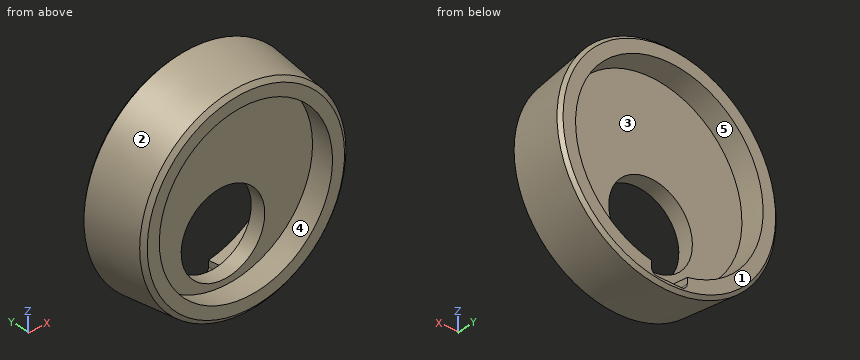
from build123d import *
from OCP.BRepFilletAPI import BRepFilletAPI_MakeChamfer

# Parameters (mm, degrees)
CUT_EXTRUDE1_DEPTH = 28.123421613
SKETCH3_R          = 2
CUT_EXTRUDE2_DEPTH = 2
SKETCH8_R          = 25.2248299
CUT_EXTRUDE4_DEPTH = 12
SKETCH11_R         = 7
CUT_EXTRUDE6_DEPTH = 27.946613887
CUT_EXTRUDE7_DEPTH = 3.6
CHAMFER1_SIZE      = 0.6
CHAMFER1_SIZE2     = 0.68091755
CHAMFER1_SIZE2_2   = 0.542425845


with BuildPart() as part:
    # Sketch1 → Revolve1 (revolve)
    with BuildSketch(Plane.XY, mode=Mode.PRIVATE) as revolve1_sk:
        Polygon((0, 0), (-17.2, 0), (-15.1, -12), (0, -12), align=None)
    revolve(revolve1_sk.sketch.rotate(Axis((0, 0, 0), (0, -1, 0)), 270), axis=Axis((0, 0, 0), (0, -1, 0)))

    # Sketch2 → Cut-Extrude1 (cut, through all)
    with BuildSketch(Plane(origin=(0, 0, 0), x_dir=(1, 0, 0), z_dir=(0, 1, 0))):
        with BuildLine():
            Line((-9.1, -5.8), (-7.3, -5.8))
            Line((-7.3, -5.8), (-7.3, -10.756858277))
            ThreePointArc((-7.3, -10.756858277), (0, -13), (7.3, -10.756858277))
            Line((7.3, -10.756858277), (7.3, -5.8))
            Line((7.3, -5.8), (9.1, -5.8))
            Line((9.1, -5.8), (9.1, -4))
            Line((9.1, -4), (7.3, -4))
            Line((7.3, -4), (7.3, 0))
            Line((7.3, 0), (13, 0))
            ThreePointArc((13, 0), (0, 13), (-13, 0))
            Line((-13, 0), (-7.3, 0))
            Line((-7.3, 0), (-7.3, -4))
            Line((-7.3, -4), (-9.1, -4))
            Line((-9.1, -4), (-9.1, -5.8))
        make_face()
    extrude(amount=-CUT_EXTRUDE1_DEPTH, mode=Mode.SUBTRACT)

    # Sketch3 → Cut-Extrude2 (cut)
    with BuildSketch(Plane(origin=(0, 0, 0), x_dir=(1, 0, 0), z_dir=(0, 1, 0))):
        with Locations((-8.1, -4.9)):
            Circle(SKETCH3_R)
        with Locations((8.1, -4.9)):
            Circle(SKETCH3_R)
    extrude(amount=-CUT_EXTRUDE2_DEPTH, mode=Mode.SUBTRACT)

    # Sketch8 → Cut-Extrude4 (cut)
    with BuildSketch(Plane.XZ.offset(12)):
        Circle(SKETCH8_R)
    extrude(amount=-CUT_EXTRUDE4_DEPTH, mode=Mode.SUBTRACT)


with BuildPart() as body_2:
    # Sketch6 → Revolve2 (revolve)
    with BuildSketch(Plane(origin=(0, 0, 0), x_dir=(0, 0, -1), z_dir=(1, 0, 0))):
        Polygon((17.2, 0), (18.4, 10.6), (15.701886792, 10.6), (15.294339623, 7), (0, 7), (0, 4.4), (15, 4.4), (14.501886792, 0), align=None)
    revolve(axis=Axis((0, 4.4, 0), (0, 1, 0)))

    # Sketch11 → Cut-Extrude6 (cut, through all)
    with BuildSketch(Plane(origin=(0, 7, 0), x_dir=(1, 0, 0), z_dir=(0, 1, 0))):
        with Locations(Location((0, 7, 0), (0, 0, 270))):
            Circle(SKETCH11_R)
    extrude(amount=-CUT_EXTRUDE6_DEPTH, mode=Mode.SUBTRACT)

    # Sketch12 → Cut-Extrude7 (cut)
    with BuildSketch(Plane(origin=(0, 10.6, 0), x_dir=(1, 0, 0), z_dir=(0, 1, 0))):
        with BuildLine():
            Line((3, 16.4), (3, 14.788468719))
            Line((3, 14.788468719), (-3, 14.788468719))
            Line((-3, 14.788468719), (-3, 16.4))
            ThreePointArc((-3, 16.4), (-2.707106781, 17.107106781), (-2, 17.4))
            Line((-2, 17.4), (2, 17.4))
            ThreePointArc((2, 17.4), (2.707106781, 17.107106781), (3, 16.4))
        make_face()
    extrude(amount=-CUT_EXTRUDE7_DEPTH, mode=Mode.SUBTRACT)

    # Chamfer1: one chamfer whose edges measure the first distance from different faces: ONE call of the kernel's chamfer builder (chamfer() names one face for all edges)
    chamfer1_edges_1 = [body_2.edges().sort_by_distance(p)[0] for p in [
        (0, 0, 17.2),
    ]]
    chamfer1_side_1 = [body_2.faces().sort_by_distance(p)[0] for p in [
        (0, 5.3, 17.8),
    ]]
    chamfer1_edges_2 = [body_2.edges().sort_by_distance(p)[0] for p in [
        (0, 10.6, 18.4),
    ]]
    chamfer1_side_2 = [body_2.faces().sort_by_distance(p)[0] for p in [
        (0, 10.6, 17.879569409),
    ]]
    chamfer1 = BRepFilletAPI_MakeChamfer(body_2.part.solid().wrapped)
    for e in chamfer1_edges_1:
        chamfer1.Add(CHAMFER1_SIZE, CHAMFER1_SIZE2, e.wrapped, chamfer1_side_1[0].wrapped)  # the first distance lies on this face
    for e in chamfer1_edges_2:
        chamfer1.Add(CHAMFER1_SIZE, CHAMFER1_SIZE2_2, e.wrapped, chamfer1_side_2[0].wrapped)  # the first distance lies on this face
    add(Compound.cast(chamfer1.Shape()), mode=Mode.REPLACE)


solid = body_2.part
Build history of the part. All positions in model axes, mm. Face numbers are marked on the shaded views. A direction names the side the tool comes from. Give positions to 0.01 mm unless a question says otherwise; leave off trailing zeros. Write each loop counter-clockwise with the first axis right and the second up, starting at its lowest first coordinate (ties: lowest second). Pieces come first, ordered by that corner, then holes. Notation, with made-up numbers: (68.5, -3) - (81.5, -3) arc R19 cw to (81.5, 23) - close; hole circle Ø1 at (60.25, 13.25). An arc over 180 degrees is marked (long way). Use one line per item in the form item = value. Start each with the question number.
1. Band-saw the part on B-B on y = 2. Write the cut outline in (x, z).
2. Band-saw the part on A-A on y = 7.5. Write the cut outline in (x, z).
3. Probe line 1 (Y direction, x = 8, z = -1); line 2 (X direction, y = 4.95, z = -7); line 3 (X direction, y = 4.75, z = -8.5). List the from-to ranges inside material, lowest first. Write a range as [from, to].
4. Drop flat-ended pins along their axis: pin 1 Ø1.8 at (x, y) = (0.5, 8.5) entering from +Z; pin 2 Ø1 at (x, y) = (-11.5, 9) entering from -Z; pin 3 Ø1.5 at (y, z) = (9.5, -15.5) entering from +X; pin 4 Ø12 at (x, z) = (11, -6.5) entering from +Y. Give the stop position or say it passes through.
5. Two-plate mould, pull along X, no slides. Class the marked faces 1, 2 and 3: released by +X, released by -X, zero draft, split by the parting line, or undercut.
6. 3-axis set-ups, long thin cutter, end or side, ignore diameter. For the marked faces 4 and 5: which of +Z, -Z, +X, -X, +Y, -Y reach the whole face in a straight line?
Conclusion:
q1.outline = circle Ø34.85 at (0, 0); hole circle Ø29.46 at (0, 0)
q2.outline = circle Ø36.1 at (0, 0); hole (-3, -16.4) arc R1 ccw to (-2, -17.4) - (2, -17.4) arc R1 ccw to (3, -16.4) - (3, -15.05) arc R15.35 ccw (long way) to (-3, -15.05) - close
q3.line_1 = [4.4, 7]
q3.line_2 = [-16.32, -7], [7, 16.32]
q3.line_3 = [-15.57, -6.84], [6.84, 15.57]
q4.pin_1 = 18.26
q4.pin_2 = -14.53
q4.pin_3 = 10.8
q4.pin_4 = 10.6
q5.face_1 = zero draft
q5.face_2 = split by the parting line
q5.face_3 = undercut
q6.face_4 = none
q6.face_5 = +Y
